Build history of the part. All positions in model axes, mm. A direction names the side the tool comes from. Give positions to 0.01 mm unless a question says otherwise; leave off trailing zeros. Loops run counter-clockwise (first coordinate to the right, second up) from the corner with the lowest first, then second, coordinate; pieces in that order, holes last. Notation, with made-up numbers: (26.25, -4) -> (69.25, -4) arc R21 cw to (69.25, 26) -> close; hole circle Ø11 at (28.25, 10.25). An arc over 180 degrees is marked (long way). One line per question, with ' | ' between items. Start each with the question number.
(1) Drill centre lines: L1, parallel to X at y = 5.5, z = 5; L2, parallel to X at y = 4.75, z = 5.5; L3, parallel to Y at x = -26, z = 2. Where is each one in solid material? Low to high. Write a range as from..to.
(2) Flat gauge pins, fed straight in: pin 1 Ø2 at (x, z) = (29, 5.5) entering from +Y; pin 2 Ø1.5 at (x, z) = (1, 9) entering from -Y. Where does each tip first touch, or does it go through?
(3) Slice it at D-D, the plane y = 0.75. Write the cut outline in (x, z), then the cut area to 3 significant figures.
(4) Mould opens along Z. For faces 1 (the face through (-35.547, 5.526, 4.489)), 2 (the face through (23.32, 0.51, 4.93)), 3 (the face through (-24.867, 5.526, 4.925)), 4 (the face through (-40.15, 5.53, 1.48)) say: pulls with the +Z half, pulls with the -Z half, needs draft (parallel to the pull), parting line crosses it, or undercut.
(5) Slice it at B-B, the plane z = 9. Write the cut outline in (x, y).
(6) Slice it at A-A, the plane z = 5. Write the cut outline in (x, y), then the cut area to 3 significant figures.
(7) Slice it at C-C, the plane x = -14.5. Write the cut outline in (y, z).
(8) 3-axis set-ups, long thin cutter, end or side, ignore diameter. For faces 5 (the face through (28, 2.498, 5)), 6 (the face through (22.331, 3, 5)), 7 (the face through (27, -0.502, 5)): which of +Z, -Z, +X, -X, +Y, -Y reach the whole face in a straight line?
```python
from build123d import *

# Parameters (mm, degrees)
BOSS_EXTRUDE1_DEPTH = 10
CHAMFER1_SIZE       = 3
CHAMFER4_SIZE       = 4
CHAMFER5_SIZE       = 2
CUT_EXTRUDE1_REACH  = 10
SKETCH4_R           = 1.7


with BuildPart() as part:
    # Sketch2 → Boss-Extrude1 (new body)
    with BuildSketch(Plane.XY):
        Polygon((-41.668551289, 7.497735583), (-41.668551289, 3.497735583), (22.331448711, 3.497735583), (22.331448711, -0.502264417), (30.331448711, -0.502264417), (30.331448711, 2.497735583), (26.331448711, 2.497735583), (26.331448711, 7.497735583), align=None)
    extrude(amount=BOSS_EXTRUDE1_DEPTH)

    # Chamfer1
    chamfer1_edges = [part.edges().sort_by_distance(p)[0] for p in [
        (-41.668551289, 5.497735583, 0),
    ]]
    chamfer(chamfer1_edges, length=CHAMFER1_SIZE)

    # Chamfer4
    chamfer4_edges = [part.edges().sort_by_distance(p)[0] for p in [
        (26.331448711, 7.497735583, 5),
    ]]
    chamfer(chamfer4_edges, length=CHAMFER4_SIZE)

    # Chamfer5
    chamfer5_edges = [part.edges().sort_by_distance(p)[0] for p in [
        (22.331448711, -0.502264417, 5),
    ]]
    chamfer(chamfer5_edges, length=CHAMFER5_SIZE)

    # Sketch4 → Cut-Extrude1 (cut, up to next)
    with BuildSketch(Plane(origin=(0, 7.497735583, 0), x_dir=(1, 0, 0), z_dir=(0, 1, 0)), mode=Mode.PRIVATE) as cut_extrude1_sk1:
        with Locations((-37.168551289, -5)):
            Circle(SKETCH4_R)
    cut_extrude1_tool1 = extrude(cut_extrude1_sk1.sketch, amount=-CUT_EXTRUDE1_REACH, mode=Mode.PRIVATE) & part.part
    add(cut_extrude1_tool1.solids().sort_by_distance((-37.168551, 7.497736, 5))[0], mode=Mode.SUBTRACT)
    # Sketch4 → Cut-Extrude1 (cut, up to next)
    with BuildSketch(Plane(origin=(0, 7.497735583, 0), x_dir=(1, 0, 0), z_dir=(0, 1, 0)), mode=Mode.PRIVATE) as cut_extrude1_sk2:
        with Locations((-23.168551289, -5)):
            Circle(SKETCH4_R)
    cut_extrude1_tool2 = extrude(cut_extrude1_sk2.sketch, amount=-CUT_EXTRUDE1_REACH, mode=Mode.PRIVATE) & part.part
    add(cut_extrude1_tool2.solids().sort_by_distance((-23.168551, 7.497736, 5))[0], mode=Mode.SUBTRACT)


solid = part.part
```
Final values:
1) L1: -41.67..-38.87, -35.47..-24.87, -21.47..24.33 | L2: -41.67..-38.79, -35.54..-24.79, -21.54..25.08 | L3: 3.5..7.5
2) pin 1: y = 2.5 | pin 2: y = 3.5
3) outline: (23.08, 0) -> (30.33, 0) -> (30.33, 10) -> (23.08, 10) -> close | area: 72.5 mm2
4) face 1: undercut | face 2: needs draft | face 3: undercut | face 4: pulls with the -Z half
5) outline: (-41.67, 3.5) -> (22.33, 3.5) -> (22.33, 1.5) -> (24.33, -0.5) -> (30.33, -0.5) -> (30.33, 2.5) -> (26.33, 2.5) -> (26.33, 3.5) -> (22.33, 7.5) -> (-41.67, 7.5) -> close
6) outline: (-41.67, 3.5) -> (-38.87, 3.5) -> (-38.87, 7.5) -> (-41.67, 7.5) -> close; (-35.47, 3.5) -> (-24.87, 3.5) -> (-24.87, 7.5) -> (-35.47, 7.5) -> close; (-21.47, 3.5) -> (22.33, 3.5) -> (22.33, 1.5) -> (24.33, -0.5) -> (30.33, -0.5) -> (30.33, 2.5) -> (26.33, 2.5) -> (26.33, 3.5) -> (22.33, 7.5) -> (-21.47, 7.5) -> close | area: 263 mm2
7) outline: (3.5, 0) -> (7.5, 0) -> (7.5, 10) -> (3.5, 10) -> close
8) face 5: +Z, -Z, +X, +Y | face 6: +Z, -Z, -X, -Y | face 7: +Z, -Z, +X, -X, -Y
